Could you check a few things on this model? Use its own coordinates, in mm. Face numbers are marked on the shaded views. A direction names the side the tool comes from. Round coordinates to 2 decimals unless told otherwise and drop trailing zeros. Loops run counter-clockwise (first coordinate to the right, second up) from the corner with the lowest first, then second, coordinate; pieces in that order, holes last. Notation, with made-up numbers: M 56.5,24.5 L 100.5,24.5 A21 cw 100.5,54.5 Z; hole C 29.5,68.25 d7. An arc over 180 degrees is marked long. One line per item, written item: value. Start each with the question number.
Q1. Which directions (+Z, -Z, +X, -X, +Y, -Y) give clear straight access to the entire face, cutting with the end or side of a thin tool? Please do the marked faces 1 and 2.
Q2. Imagine slicing it at B-B (y = 8). Please give me the cut outline in (x, z).
Q3. Imagine slicing it at D-D (y = 0). Give the number of separate pieces and of enclosed holes in the cut face, then the cut area to 3 significant figures.
Q4. Imagine slicing it at C-C (z = 8). Please give me the cut outline in (x, y), then the cut area to 3 significant figures.
Q5. Imagine slicing it at A-A (x = 22). Please give me the cut outline in (y, z).
Q6. Please list where these lines run through material, in increasing order: line 1 along Z through (x, y) = (6.63, 33.5); line 2 along X through (y, z) = (6.5, -1); line 3 along Y through (x, z) = (23, -12).
Q7. I'm going to push flat-ended pins straight in: pin 1 Ø1.8 at (y, z) = (0, 8) entering from -X; pin 2 Ø4 at (y, z) = (-2, 0) entering from -X; pin 3 Ø17.5 at (x, z) = (13.5, 5.5) entering from -Y. Where does each tip first touch, or does it pass through?
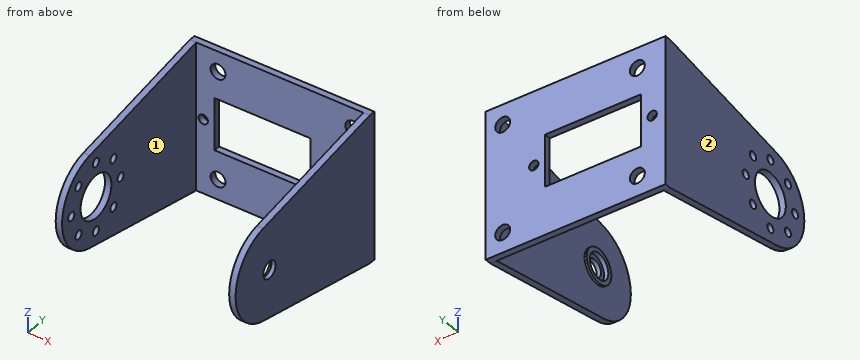
from build123d import *

# Parameters (mm, degrees)
SKETCH2_W           = 34.6
SKETCH2_H           = 1.5
SKETCH2_R           = 11
SKETCH2_R_2         = 1
SKETCH2_R_3         = 5
BOSS_EXTRUDE1_DEPTH = 1.5
SKETCH2_3_W         = 34.6
SKETCH2_3_H         = 1.5
BOSS_EXTRUDE2_DEPTH = 40.75
BOSS_EXTRUDE3_START = 40.75
SKETCH2_6_W         = 34.6
SKETCH2_6_H         = 1.5
SKETCH2_6_R         = 11
SKETCH2_6_R_2       = 1
SKETCH2_6_R_3       = 5
SKETCH2_6_R_4       = 4
SKETCH2_6_R_5       = 3
BOSS_EXTRUDE3_DEPTH = 1.5
SKETCH3_R           = 1.1
SKETCH3_R_2         = 1.75
SKETCH3_W           = 22.5
SKETCH3_H           = 12.2
CUT_EXTRUDE1_DEPTH  = 46
BOSS_EXTRUDE4_START = 40.75
SKETCH2_7_R         = 4
SKETCH2_7_R_2       = 3
BOSS_EXTRUDE4_DEPTH = 0.5
SKETCH4_R           = 3
SKETCH4_R_2         = 2
BOSS_EXTRUDE5_DEPTH = 1


with BuildPart() as part:
    # Sketch2 → Boss-Extrude1 (new body)
    with BuildSketch(Plane(origin=(0, 0, 0), x_dir=(0, 0, -1), z_dir=(1, 0, 0))):
        with BuildLine():
            Line((17.3, 32.5), (-17.3, 32.5))
            Line((-17.3, 32.5), (-10.810767407, -2.031577728))
            ThreePointArc((-10.810767407, -2.031577728), (-1.020185895, 10.952589682), (11, 0))
            ThreePointArc((11, 0), (10.952589682, -1.020185895), (10.810767407, -2.031577728))
            Line((10.810767407, -2.031577728), (17.3, 32.5))
        make_face()
        with Locations((0, 33.25)):
            Rectangle(SKETCH2_W, SKETCH2_H)
        Circle(SKETCH2_R)
        with Locations((-5.656854249, 5.656854249)):
            Circle(SKETCH2_R_2, mode=Mode.SUBTRACT)
        with Locations((-8, 0)):
            Circle(SKETCH2_R_2, mode=Mode.SUBTRACT)
        with Locations((-5.656854249, -5.656854249)):
            Circle(SKETCH2_R_2, mode=Mode.SUBTRACT)
        with Locations((0, -8)):
            Circle(SKETCH2_R_2, mode=Mode.SUBTRACT)
        with Locations((5.656854249, -5.656854249)):
            Circle(SKETCH2_R_2, mode=Mode.SUBTRACT)
        with Locations((8, 0)):
            Circle(SKETCH2_R_2, mode=Mode.SUBTRACT)
        with Locations((5.656854249, 5.656854249)):
            Circle(SKETCH2_R_2, mode=Mode.SUBTRACT)
        with Locations((0, 8)):
            Circle(SKETCH2_R_2, mode=Mode.SUBTRACT)
        Circle(SKETCH2_R_3, mode=Mode.SUBTRACT)
    extrude(amount=BOSS_EXTRUDE1_DEPTH)

    # Sketch2<3> → Boss-Extrude2 (add)
    with BuildSketch(Plane(origin=(0, 0, 0), x_dir=(0, 0, -1), z_dir=(1, 0, 0))):
        with Locations((0, 33.25)):
            Rectangle(SKETCH2_3_W, SKETCH2_3_H)
    extrude(amount=BOSS_EXTRUDE2_DEPTH)

    # Sketch2<6> → Boss-Extrude3 (add)
    with BuildSketch(Plane(origin=(0, 0, 0), x_dir=(0, 0, -1), z_dir=(1, 0, 0)).offset(BOSS_EXTRUDE3_START)):
        with Locations((0, 33.25)):
            Rectangle(SKETCH2_6_W, SKETCH2_6_H)
        with BuildLine():
            Line((17.3, 32.5), (-17.3, 32.5))
            Line((-17.3, 32.5), (-10.810767407, -2.031577728))
            ThreePointArc((-10.810767407, -2.031577728), (-1.020185895, 10.952589682), (11, 0))
            ThreePointArc((11, 0), (10.952589682, -1.020185895), (10.810767407, -2.031577728))
            Line((10.810767407, -2.031577728), (17.3, 32.5))
        make_face()
        Circle(SKETCH2_6_R)
        with Locations((-5.656854249, 5.656854249)):
            Circle(SKETCH2_6_R_2, mode=Mode.SUBTRACT)
        with Locations((-8, 0)):
            Circle(SKETCH2_6_R_2, mode=Mode.SUBTRACT)
        with Locations((-5.656854249, -5.656854249)):
            Circle(SKETCH2_6_R_2, mode=Mode.SUBTRACT)
        with Locations((0, -8)):
            Circle(SKETCH2_6_R_2, mode=Mode.SUBTRACT)
        with Locations((5.656854249, -5.656854249)):
            Circle(SKETCH2_6_R_2, mode=Mode.SUBTRACT)
        with Locations((8, 0)):
            Circle(SKETCH2_6_R_2, mode=Mode.SUBTRACT)
        with Locations((5.656854249, 5.656854249)):
            Circle(SKETCH2_6_R_2, mode=Mode.SUBTRACT)
        with Locations((0, 8)):
            Circle(SKETCH2_6_R_2, mode=Mode.SUBTRACT)
        Circle(SKETCH2_6_R_3, mode=Mode.SUBTRACT)
        with Locations((0, 8)):
            Circle(SKETCH2_6_R_2)
        with Locations((-5.656854249, 5.656854249)):
            Circle(SKETCH2_6_R_2)
        with Locations((-8, 0)):
            Circle(SKETCH2_6_R_2)
        with Locations((-5.656854249, -5.656854249)):
            Circle(SKETCH2_6_R_2)
        with Locations((0, -8)):
            Circle(SKETCH2_6_R_2)
        with Locations((5.656854249, -5.656854249)):
            Circle(SKETCH2_6_R_2)
        with Locations((8, 0)):
            Circle(SKETCH2_6_R_2)
        with Locations((5.656854249, 5.656854249)):
            Circle(SKETCH2_6_R_2)
        Circle(SKETCH2_6_R_3)
        Circle(SKETCH2_6_R_4, mode=Mode.SUBTRACT)
        Circle(SKETCH2_6_R_4)
        Circle(SKETCH2_6_R_5, mode=Mode.SUBTRACT)
    extrude(amount=BOSS_EXTRUDE3_DEPTH)

    # Sketch3 → Cut-Extrude1 (cut, through all)
    with BuildSketch(Plane(origin=(0, 34, 0), x_dir=(1, 0, 0), z_dir=(0, 1, 0))):
        with Locations((30.945, 0)):
            Circle(SKETCH3_R)
        with Locations((3.145, 0)):
            Circle(SKETCH3_R)
        with Locations((6.63, 12.583801515)):
            Circle(SKETCH3_R_2)
        with Locations((38.257478, 12.583801515)):
            Circle(SKETCH3_R_2)
        with Locations((38.257478, -12.583801515)):
            Circle(SKETCH3_R_2)
        with Locations((6.63, -12.583801515)):
            Circle(SKETCH3_R_2)
        with Locations((17.045, 0)):
            Rectangle(SKETCH3_W, SKETCH3_H)
    extrude(amount=-CUT_EXTRUDE1_DEPTH, mode=Mode.SUBTRACT)

    # Sketch2<7> → Boss-Extrude4 (add)
    with BuildSketch(Plane(origin=(0, 0, 0), x_dir=(0, 0, -1), z_dir=(1, 0, 0)).offset(BOSS_EXTRUDE4_START)):
        Circle(SKETCH2_7_R)
        Circle(SKETCH2_7_R_2, mode=Mode.SUBTRACT)
    extrude(amount=-BOSS_EXTRUDE4_DEPTH)

    # Sketch4 → Boss-Extrude5 (add)
    with BuildSketch(Plane(origin=(42.25, 0, 0), x_dir=(0, 0, -1), z_dir=(1, 0, 0))):
        Circle(SKETCH4_R)
        Circle(SKETCH4_R_2, mode=Mode.SUBTRACT)
    extrude(amount=-BOSS_EXTRUDE5_DEPTH)


solid = part.part
Report:
1. face 1: +Z, -Z, -Y
1. face 2: +Z, -Z, -X, +Y, -Y
2. outline: M 0,-12.7 L 1.5,-12.7 L 1.5,-1 L 0,-1 Z; M 0,1 L 1.5,1 L 1.5,12.7 L 0,12.7 Z; M 40.75,-12.7 L 42.25,-12.7 L 42.25,12.7 L 40.75,12.7 Z
3. separate pieces: 6
3. enclosed holes: 0
3. area: 40.2 mm²
4. outline: M 0,-7.55 L 1.5,-7.55 L 1.5,-1 L 0,-1 Z; M 0,1 L 1.5,1 L 1.5,32.5 L 40.75,32.5 L 40.75,-7.55 L 42.25,-7.55 L 42.25,34 L 0,34 Z
4. area: 181 mm²
5. outline: M 32.5,-17.3 L 34,-17.3 L 34,-6.1 L 32.5,-6.1 Z; M 32.5,6.1 L 34,6.1 L 34,17.3 L 32.5,17.3 Z
6. line 1: z = -17.3 to -14.33, -10.83 to -6.1, 6.1 to 10.83, 14.33 to 17.3
6. line 2: x = 0 to 1.5, 40.75 to 42.25
6. line 3: y = 32.5 to 34
7. pin 1: stops at x = 40.75
7. pin 2: stops at x = 40.25
7. pin 3: stops at y = 32.5
